Could you check a few things on this model? Use its own coordinates, in mm. A direction names the side the tool comes from. Give positions to 0.01 mm unless a question says otherwise; leave off trailing zeros. Write each loop counter-clockwise with the first axis right and the second up, starting at its lowest first coordinate (ties: lowest second). Pieces come first, ordered by that corner, then holes. Notation, with made-up numbers: M 31,49.25 L 43,49.25 A13 ccw 43,65.25 Z; hole C -30.75,75 d3. An arc over 180 degrees is marked long. One line per item, written item: value.
```python
from build123d import *

# Parameters (mm, degrees)
SKETCH1_R           = 42.5
SKETCH1_R_2         = 37.5
BOSS_EXTRUDE1_DEPTH = 10
SKETCH2_R           = 39.5
SKETCH2_R_2         = 37.5
BOSS_EXTRUDE2_DEPTH = 50
SKETCH3_R           = 39.5
BOSS_EXTRUDE3_DEPTH = 2
FILLET1_R           = 1
CUT_EXTRUDE1_DEPTH  = 100


with BuildPart() as part:
    # Sketch1 → Boss-Extrude1 (new body)
    with BuildSketch(Plane.XY):
        Circle(SKETCH1_R)
        Circle(SKETCH1_R_2, mode=Mode.SUBTRACT)
    extrude(amount=BOSS_EXTRUDE1_DEPTH)

    # Sketch2 → Boss-Extrude2 (add)
    with BuildSketch(Plane.XY.offset(10)):
        Circle(SKETCH2_R)
        Circle(SKETCH2_R_2, mode=Mode.SUBTRACT)
    extrude(amount=BOSS_EXTRUDE2_DEPTH)

    # Sketch3 → Boss-Extrude3 (add)
    with BuildSketch(Plane.XY.offset(60)):
        Circle(SKETCH3_R)
    extrude(amount=BOSS_EXTRUDE3_DEPTH)

    # Fillet1
    fillet1_edges = [part.edges().sort_by_distance(p)[0] for p in [
        (-39.5, 0, 62),
    ]]
    fillet(fillet1_edges, radius=FILLET1_R)

    # Sketch4 → Cut-Extrude1 (cut)
    with BuildSketch(Plane.XY.offset(62)):
        with BuildLine():
            ThreePointArc((0, -25.004064668), (-3, -28.004064668), (0, -31.004064668))
            Line((0, -31.004064668), (0, -25.004064668))
        make_face()
        with BuildLine():
            Line((0, -25.004064668), (0, -31.004064668))
            ThreePointArc((0, -31.004064668), (2.121320344, -30.125385012), (3, -28.004064668))
            ThreePointArc((3, -28.004064668), (2.121320344, -25.882744324), (0, -25.004064668))
        make_face()
    extrude(amount=-CUT_EXTRUDE1_DEPTH, mode=Mode.SUBTRACT)


solid = part.part
```
1) If we section it at B-B, the plane z = 33: Write out the boundary of the cut face in (x, y), then the cut area to 3 significant figures.
Outcome:
outline: C 0,0 d79; hole C 0,0 d75
area: 484 mm^2
2) I'm going to push flat-ended pins straight in: pin 1 (3 mm diameter, centred on x = 31.5, z = 46, fed in from -Y); pin 2 (10 mm diameter, centred on x = 18.5, y = 15.5, fed in from -Z); pin 3 (5 mm diameter, centred on y = 27.5, z = 16, fed in from +X). Where does each tip first touch, or does it pass through?
Outcome:
pin 1: stops at y = -25.7
pin 2: stops at z = 60
pin 3: stops at x = 30.58
3) Please list where these lines run through material, in increasing order: L1, parallel to Y at x = 0, z = 15.5; L2, parallel to Z at x = 34.5, y = 8; L3, parallel to X at y = 15, z = 6. Write a range as from..to.
Outcome:
L1: y = -39.5..-37.5, 37.5..39.5
L2: z = 60..62
L3: x = -39.76..-34.37, 34.37..39.76
4) If we section it at C-C, the plane z = 8.5: Write out the boundary of the cut face in (x, y).
Outcome:
outline: C 0,0 d85; hole C 0,0 d75
5) If we section it at A-A, the plane y = 0: Write out the boundary of the cut face in (x, z).
Outcome:
outline: M -42.5,0 L -37.5,0 L -37.5,60 L 37.5,60 L 37.5,0 L 42.5,0 L 42.5,10 L 39.5,10 L 39.5,61 A1 ccw 38.5,62 L -38.5,62 A1 ccw -39.5,61 L -39.5,10 L -42.5,10 Z
6) On a 3-axis mill with a long thin cutter (end or side, diameter ignored), from which of +Z, -Z, +X, -X, +Y, -Y can I reach the whole of each face in a straight line? I mean faces 1 (the face through (-1, 1, 62)), 2 (the face through (-4.88, 37.18, 29.58)). Say none if no direction works.
Outcome:
face 1: +Z, +X, -X, +Y, -Y
face 2: -Z
7) We'd pull the mould along Y, two halves only. Please class faces 3 (the face through (-29.11, 26.7, 35.14)), 4 (the face through (38, -12, 10)), 5 (the face through (-1, 1, 60)): pulls with the +Y half, pulls with the -Y half, needs draft (parallel to the pull), parting line crosses it, or undercut.
Outcome:
face 3: parting line crosses it
face 4: needs draft
face 5: undercut
